from build123d import *

# Parameters (mm, degrees)
SKETCH1_W           = 60
SKETCH1_H           = 250
SKETCH1_R           = 1.6
BOSS_EXTRUDE1_DEPTH = 10


with BuildPart() as part:
    # Sketch1 → Boss-Extrude1 (new body)
    with BuildSketch(Plane(origin=(0, 0, 0), x_dir=(1, 0, 0), z_dir=(0, 1, 0))):
        with Locations((30, -125)):
            Rectangle(SKETCH1_W, SKETCH1_H)
        with Locations(Location((30, -170, 0), (0, 0, 270))):
            Circle(SKETCH1_R, mode=Mode.SUBTRACT)
        Polygon((20, -215), (20, -235), (40, -235), (40, -225), (30, -225), (30, -215), align=None, mode=Mode.SUBTRACT)
    extrude(amount=BOSS_EXTRUDE1_DEPTH)


solid = part.part
The model under review builds one solid part; all positions refer to its coordinate system, in mm. A direction names the side the tool comes from. Round coordinates to 2 decimals unless told otherwise and drop trailing zeros. Loops run counter-clockwise (first coordinate to the right, second up) from the corner with the lowest first, then second, coordinate; pieces in that order, holes last. Notation, with made-up numbers: (35, -32.75) - (57, -32.75) arc R25 cw to (57, -19.75) - close; hole circle Ø2 at (-26.5, 7.5). An arc over 180 degrees is marked (long way). Use CSV: the item, a comma, the result in double quotes.
(1) For line 1 (X direction, y = 3.5, z = 170); line 2 (X direction, y = 3, z = 216); line 3 (Z direction, x = 21, y = 8), list the stretches that pass through material, from the lowest coordinate up.
Working result:
line 1,"x = 0 to 28.4, 31.6 to 60"
line 2,"x = 0 to 20, 30 to 60"
line 3,"z = 0 to 215, 235 to 250"
(2) Clearance check with a flat-ended pin moving along its axis: P1, Ø5, axis at x = 30, z = 170, coming from the -Y side. State where the tip first meets the part, or that it passes through.
Working result:
P1,"stops at y = 0"
(3) Take a section at B-B, the plane y = 7.5. Give the boundary of the cut face in (x, z), plus the area to 3 significant figures.
Working result:
outline,"(0, 0) - (60, 0) - (60, 250) - (0, 250) - close; hole (20, 215) - (30, 215) - (30, 225) - (40, 225) - (40, 235) - (20, 235) - close; hole circle Ø3.2 at (30, 170)"
area,"14,700 mm^2"
(4) Machinability: for faces 5 (the flat face through (60, 5, 127)), 6 (the flat face through (30, 5, 235)), which of the approach directions +Z, -Z, +X, -X, +Y, -Y give a long, thin tool a straight path to every point of the face, cutting with its end or side? Answer none if there is none.
Working result:
face 5,"+Z, -Z, +X, +Y, -Y"
face 6,"+Y, -Y"
(5) The part is to be moulded in two halves that separate along Z. For faces 1 (the flat face through (40, 5, 230)), 2 (the flat face through (30, 5, 220)), 3 (the flat face through (30, 5, 0)), 4 (the flat face through (30, 10, 123)), say which applies: pulls with the +Z half, pulls with the -Z half, needs draft (parallel to the pull), parting line crosses it, or undercut.
Working result:
face 1,"undercut"
face 2,"undercut"
face 3,"pulls with the -Z half"
face 4,"needs draft"
(6) Take a section at A-A, the plane x = 34. Give the boundary of the cut face in (y, z).
Working result:
outline,"(0, 0) - (10, 0) - (10, 225) - (0, 225) - close; (0, 235) - (10, 235) - (10, 250) - (0, 250) - close"
